Print and shaded views of the part. All mm, measured from the part's lowest x, y and z. A direction names the side the tool comes from. Coordinates: 2 decimals unless noted, no trailing zeros. Order: outer loops, then holes, each group sorted by start corner. A loop starts at its lowest first (then second) coordinate and runs counter-clockwise, first axis right, second up. Notation, with made-up numbers: M -35,-8 L -28,-8 A24 ccw -28,7 Z; hole C 31.25,33.25 d7. An arc over 180 degrees is marked long. One line per item, written item: value.
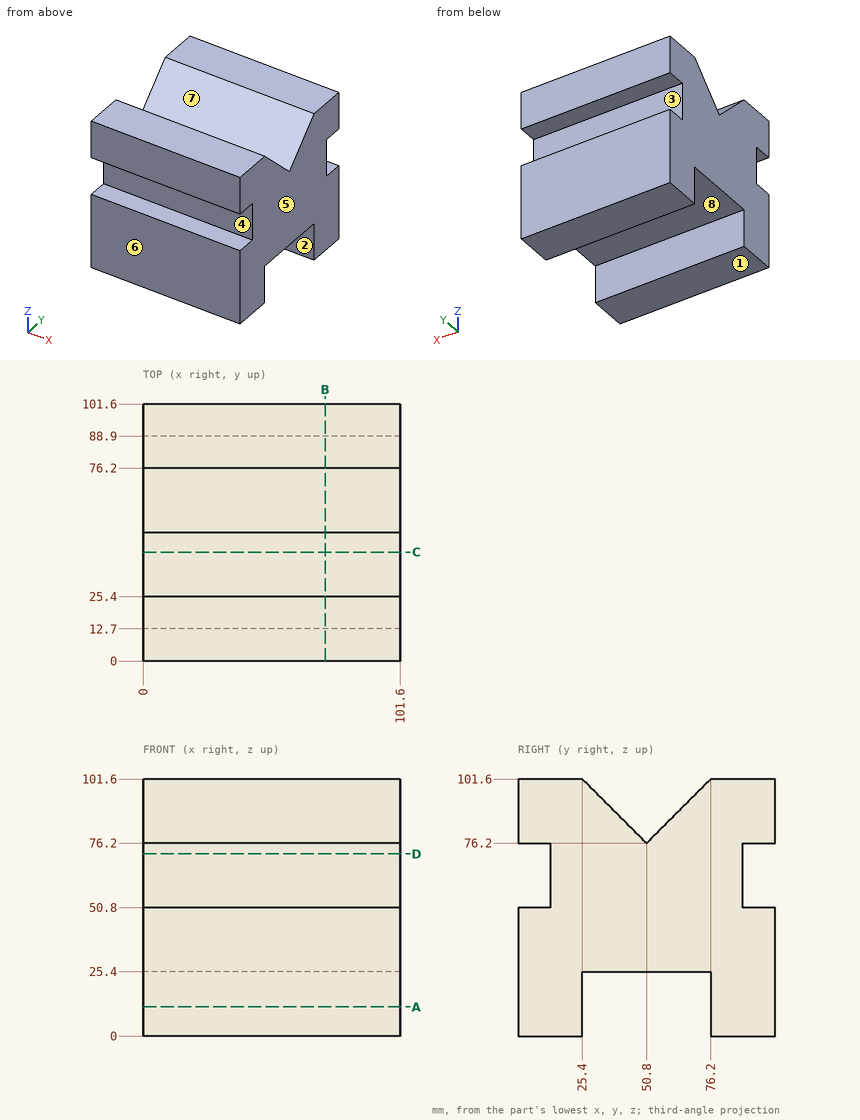
Q1. Slice it at D-D (z = 72). List the corners of the cut face in (x, y), plus the area to 3 significant figures.
Recorded:
outline: M 0,12.7 L 101.6,12.7 L 101.6,88.9 L 0,88.9 Z
area: 7,740 mm^2
Q2. Slice it at A-A (z = 11.5). List the corners of the cut face in (x, y).
Recorded:
outline: M 0,0 L 101.6,0 L 101.6,25.4 L 0,25.4 Z; M 0,76.2 L 101.6,76.2 L 101.6,101.6 L 0,101.6 Z
Q3. Slice it at C-C (y = 43). List the corners of the cut face in (x, z), plus the area to 3 significant figures.
Recorded:
outline: M 0,25.4 L 101.6,25.4 L 101.6,84 L 0,84 Z
area: 5,950 mm^2
Q4. Drill centre lines: line 1 along Y through (x, z) = (48.5, 19.5); line 2 along Z through (x, y) = (53, 89); line 3 along Y through (x, z) = (12, 75). Where is each one in solid material? Low to high.
Recorded:
line 1: y = 0 to 25.4, 76.2 to 101.6
line 2: z = 0 to 50.8, 76.2 to 101.6
line 3: y = 12.7 to 88.9
Q5. Which spindle directions (+Z, -Z, +X, -X, +Y, -Y) get a long thin tool onto all of the face, cutting with end or side? Do the marked faces 4, 5, 6, 7 and 8. Say none if no direction does.
Recorded:
face 4: +X, -X, -Y
face 5: +Z, -Z, +X, +Y, -Y
face 6: +Z, -Z, +X, -X, -Y
face 7: +Z, +X, -X
face 8: -Z, +X, -X
Q6. Pin check, flat tips, straight feed: pin 1 Ø8 at (y, z) = (40, 89.5) entering from -X; pin 2 Ø5 at (x, y) = (89, 48) entering from -Z; pin 3 Ø3 at (x, y) = (50, 43.5) entering from +Z; pin 4 Ø7.5 at (x, z) = (30.5, 66) entering from +Y. Stop position of each tip, or through.
Recorded:
pin 1: stops at x = 0
pin 2: stops at z = 25.4
pin 3: stops at z = 85
pin 4: stops at y = 88.9
Q7. Slice it at B-B (x = 72). List the corners of the cut face in (y, z).
Recorded:
outline: M 0,0 L 25.4,0 L 25.4,25.4 L 76.2,25.4 L 76.2,0 L 101.6,0 L 101.6,50.8 L 88.9,50.8 L 88.9,76.2 L 101.6,76.2 L 101.6,101.6 L 76.2,101.6 L 50.8,76.2 L 25.4,101.6 L 0,101.6 L 0,76.2 L 12.7,76.2 L 12.7,50.8 L 0,50.8 Z
Q8. Mould opens along Z. For the marked faces 1, 2 and 3 say: released by +Z, released by -Z, zero draft, split by the parting line, or undercut.
Recorded:
face 1: released by -Z
face 2: zero draft
face 3: undercut
